from build123d import *


with BuildPart() as f1:
    # F0 (on Top) → F1 (revolve)
    with BuildSketch(Plane.XY):
        Polygon((4, -36), (4, -24), (14, -14), (24, -24), (24, -36), (28, -36), (28, 0), (24, 0), (14, -10), (4, 0), (0, 0), (0, -36), align=None)
        Polygon((10.343146, -12), (4, -18.343146), (4, -5.656854), align=None, mode=Mode.SUBTRACT)
        Polygon((24, -18.343146), (17.656854, -12), (24, -5.656854), align=None, mode=Mode.SUBTRACT)
    revolve(axis=Axis((0, -18, 0), (0, -1, 0)))


solid = f1.part
Could you check a few things on this model? Use its own coordinates, in mm. A direction names the side the tool comes from. Give positions to 0.01 mm unless a question says otherwise; leave off trailing zeros. Order: outer loops, then holes, each group sorted by start corner. A loop starts at its lowest first (then second) coordinate and runs counter-clockwise, first axis right, second up.
1. I need wall thicknesses on L1, parallel to Z at x = 0, y = -32.75; L2, parallel to X at y = -34, z = 3; L3, parallel to X at y = -13.5, z = 16.5. Which ranges of each line are inside material? Lowest first, please.
Answers below:
L1: z = -28 to -24, -4 to 4, 24 to 28
L2: x = -27.84 to -23.81, -2.65 to 2.65, 23.81 to 27.84
L3: x = -22.62 to -17.43, -9.73 to 9.73, 17.43 to 22.62
2. Thinking about a two-plate mould opening in Z: for faces 4 (the flat face through (21, 0, 13)), 5 (the cylindrical face through (25.865, -17.748, -10.724)), 6 (the cylindrical face through (-23.977, -30.084, 1.055)), which applies, +Z half, -Z half, draft (parallel to the pull), parting line (faces both ways), or undercut?
Answers below:
face 4: draft
face 5: parting line
face 6: undercut
3. Which directions (+Z, -Z, +X, -X, +Y, -Y) give clear straight access to the entire face, cutting with the end or side of a thin tool? Please do faces 1 (the conical face through (-0.972, -0.486, -4.379)), 2 (the conical face through (-0.934, -18.035, -4.206)), 3 (the cylindrical face through (-0.867, -29.916, -3.905)).
Answers below:
face 1: +Y
face 2: none
face 3: -Y
4. For pin 1 (5 mm diameter, centred on y = -22.5, z = 3.5, fed in from -X); pin 2 (10 mm diameter, centred on y = -12, z = 21, fed in from -X); pin 3 (5 mm diameter, centred on x = -0.5, z = -9.5, fed in from +Y), each with a flat end and sliding along its axis, tell me the tip position at first contact or that it passes through.
Answers below:
pin 1: stops at x = -27.98
pin 2: stops at x = -22.98
pin 3: stops at y = -3.01
5. Suppose I cut it at C-C (y = -15.5). Write out the boundary of the cut face in (x, z).
Answers below:
outline: circle Ø56 at (0, 0); circle Ø42.31 at (0, 0); circle Ø25 at (0, 0); circle Ø8 at (0, 0); hole circle Ø48 at (0, 0); hole circle Ø31 at (0, 0); hole circle Ø13.69 at (0, 0)
6. Suppose I cut it at B-B (z = 0). State how many separate pieces and enclosed holes the cut face has, plus the area to 3 significant figures.
Answers below:
separate pieces: 1
enclosed holes: 4
area: 975 mm2
7. Suppose I cut it at A-A (y = -30.5). Write out the boundary of the cut face in (x, z).
Answers below:
outline: circle Ø56 at (0, 0); circle Ø8 at (0, 0); hole circle Ø48 at (0, 0)
